Study the drawing (mm; zero at the part's minimum x, y, z) and answer. A direction names the side the tool comes from. Give positions to 0.01 mm unless a question says otherwise; leave off trailing zeros. Write each loop counter-clockwise with the first axis right and the second up, starting at its lowest first coordinate (ties: lowest second). Pieces come first, ordered by that corner, then holes. Notation, with made-up numbers: (85.25, 27.5) - (132.25, 27.5) arc R17 ccw to (132.25, 33.5) - close; hole circle Ø2 at (71.25, 45). An arc over 180 degrees is marked (long way). Write each question's results on one line, items separated by ' | '. Start each with the question number.
Q1. Section C-C (y = 57.5) is taken. Determine the outline of the cut face in (x, z).
Q2. Find the intervals of material crossed by probe 1 along X at (y, z) = (25.75, 17.5); probe 2 along Y at (x, z) = (27, 17.5); probe 3 along X at (y, z) = (17, 17.5), in increasing order.
Q3. For a pull along Y with two mould halves and no side action, classify the marked faces 4, 5 and 6 as pulls with the +Y half, pulls with the -Y half, needs draft (parallel to the pull), parting line crosses it, or undercut.
Q4. Flat-ended cylindrical pins translate along their axes: pin 1 Ø10 at (x, y) = (7, 5.5) entering from +Z; pin 2 Ø2.5 at (x, z) = (6, 21) entering from +Y; pin 3 Ø6 at (x, y) = (25, 12.5) entering from -Z. Find the tip coordinate at first contact, or state that the pin passes through.
Q5. Section D-D (z = 11) is taken. Determine the outline of the cut face in (x, y).
Q6. Section A-A (x = 22.5) is taken. Determine the outline of the cut face in (y, z).
Q7. For the marked faces 1, 2 and 3, determine the directions among +Z, -Z, +X, -X, +Y, -Y from which every point of the face is accessible in a straight line to the end or side of a thin tool.
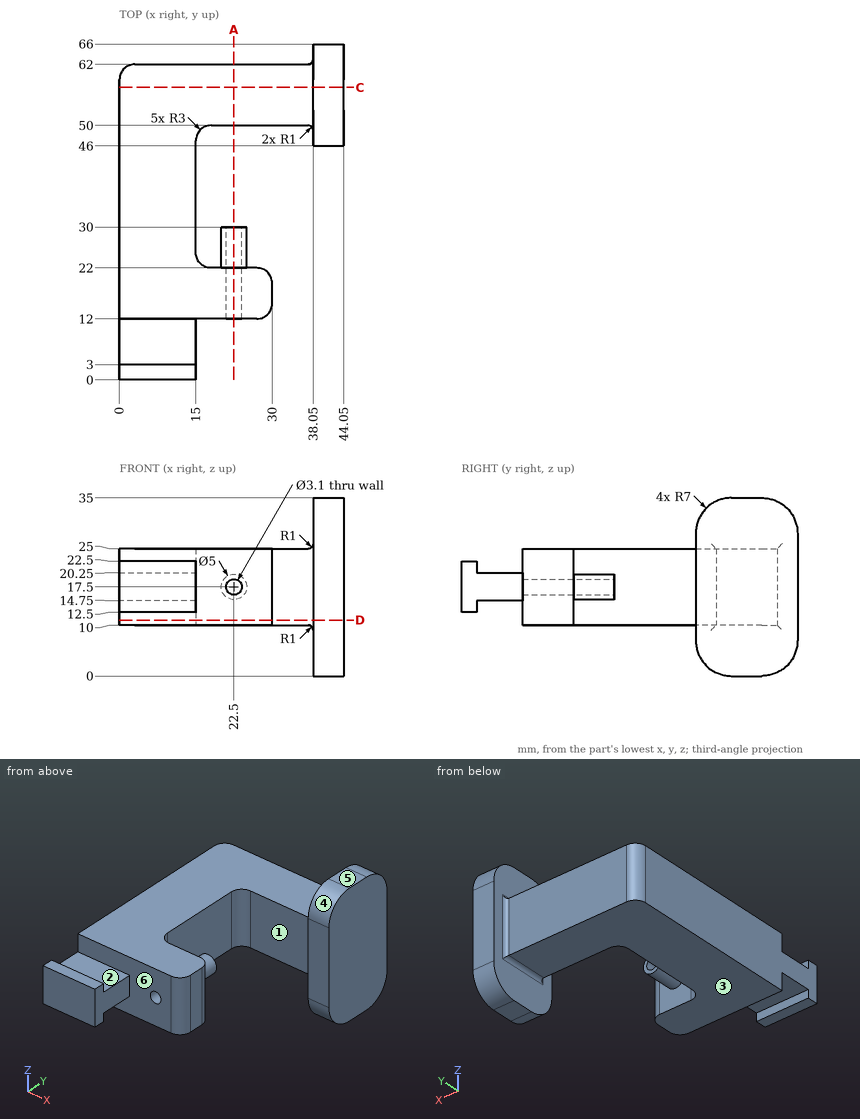
Answers below:
1) outline: (0, 10) - (37.05, 10) arc R1 cw to (38.05, 9) - (38.05, 0) - (44.05, 0) - (44.05, 35) - (38.05, 35) - (38.05, 26) arc R1 cw to (37.05, 25) - (0, 25) - close
2) probe 1: x = 0 to 15, 20 to 20.95, 24.05 to 25 | probe 2: y = 12 to 22, 50 to 62 | probe 3: x = 0 to 20.95, 24.05 to 30
3) face 4: pulls with the -Y half | face 5: needs draft | face 6: undercut
4) pin 1: stops at z = 22.5 | pin 2: stops at y = 62 | pin 3: stops at z = 10
5) outline: (0, 12) - (27, 12) arc R3 ccw to (30, 15) - (30, 19) arc R3 ccw to (27, 22) - (18, 22) arc R3 cw to (15, 25) - (15, 47) arc R3 cw to (18, 50) - (37.05, 50) arc R1 cw to (38.05, 49) - (38.05, 46) - (44.05, 46) - (44.05, 66) - (38.05, 66) - (38.05, 63) arc R1 cw to (37.05, 62) - (3, 62) arc R3 ccw to (0, 59) - close
6) outline: (12, 10) - (22, 10) - (22, 15) - (30, 15) - (30, 15.95) - (12, 15.95) - close; (12, 19.05) - (30, 19.05) - (30, 20) - (22, 20) - (22, 25) - (12, 25) - close; (50, 10) - (62, 10) - (62, 25) - (50, 25) - close
7) face 1: +Z, -Z | face 2: +Z, +X, -X | face 3: -Z, -X, +Y, -Y
